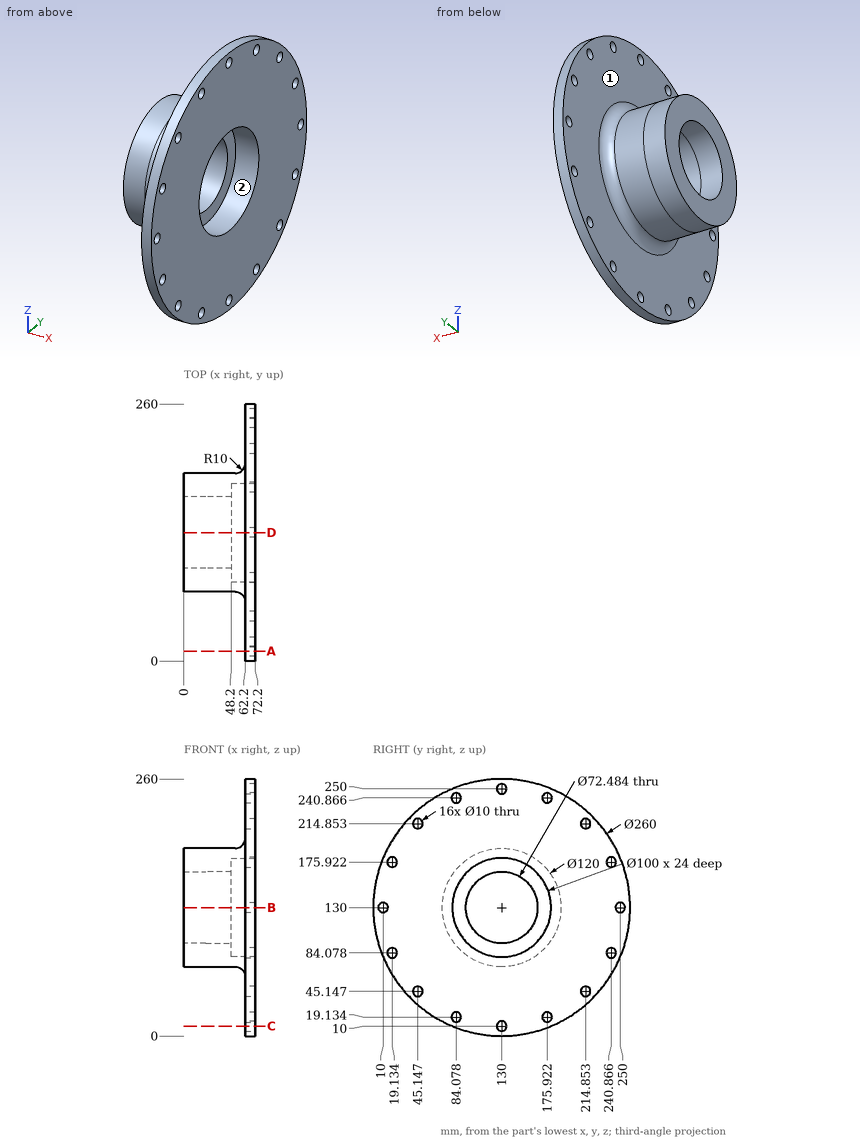
Geometry: see drawing. Coordinates: mm, zero at the bounding-box minimum. Give positions to 0.01 mm unless a question says otherwise; leave off trailing zeros. Write each loop counter-clockwise with the first axis right and the second up, starting at its lowest first coordinate (ties: lowest second). Pieces come first, ordered by that corner, then holes. Notation, with made-up numbers: M 83,58.25 L 112,58.25 A15 cw 112,69.25 Z; hole C 19,-5.75 d4. An arc over 180 degrees is marked long. Answer as a JSON object with one key per item and string values.
Q1. Cut plane A-A, the plane y = 10. Return the cut outline in (x, z).
Geometry check:
{"outline": "M 62.2,80 L 72.2,80 L 72.2,125 L 62.2,125 Z; M 62.2,135 L 72.2,135 L 72.2,180 L 62.2,180 Z"}
Q2. Contact query for flat-ended pins moving along their axis: P1, Ø3, axis at x = 15, y = 104, coming from the -Z side; P2, Ø6, axis at y = 175.92, z = 240.87, coming from the +X side; P3, Ø5, axis at y = 81, z = 193, coming from the -X side; P4, Ø6, axis at y = 188, z = 119, coming from the -X side. Output: stop coordinate, or through.
Geometry check:
{"P1": "stops at z = 75.23", "P2": "passes through", "P3": "stops at x = 62.2", "P4": "stops at x = 0"}
Q3. Mould query, pull axis Z, two halves, no side actions, for the marked faces 1 and 2. Classes: +Z half, -Z half, draft (parallel to the pull), parting line (faces both ways), or undercut.
Geometry check:
{"face 1": "draft", "face 2": "undercut"}
Q4. Ray query, line 1 along Y through (x, z) = (64.75, 130); line 2 along Y through (x, z) = (5.5, 130); line 3 along X through (y, z) = (224.5, 156). Return the intervals inside material, ascending.
Geometry check:
{"line 1": "y = 0 to 5, 15 to 80, 180 to 245, 255 to 260", "line 2": "y = 70 to 93.76, 166.24 to 190", "line 3": "x = 62.2 to 72.2"}
Q5. Cut plane B-B, the plane z = 130. Return the cut outline in (x, y).
Geometry check:
{"outline": "M 0,70 L 52.2,70 A10 cw 62.2,60 L 62.2,15 L 72.2,15 L 72.2,80 L 48.2,80 L 48.2,93.76 L 0,93.76 Z; M 0,166.24 L 48.2,166.24 L 48.2,180 L 72.2,180 L 72.2,245 L 62.2,245 L 62.2,200 A10 cw 52.2,190 L 0,190 Z; M 62.2,0 L 72.2,0 L 72.2,5 L 62.2,5 Z; M 62.2,255 L 72.2,255 L 72.2,260 L 62.2,260 Z"}
